Input: part model. Units: mm. Frame: model coordinates. Face numbers are marked on the shaded views. A direction names the side the tool comes from. Give positions to 0.01 mm unless a question says otherwise; leave off trailing zeros. Order: outer loops, then holes, each group sorted by start corner. A loop starts at its lowest first (then second) coordinate and runs counter-clockwise, first axis right, second up. Notation, with made-up numbers: (-4, 57) - (12, 57) arc R31 ccw to (12, 90) - close; hole circle Ø9 at (12.25, 57). An arc over 180 degrees is marked (long way). Answer in a Markdown table with one row per item. Add a question column.
1. Section query D-D on y = -0.4. Return loops of the section in (x, z), and give its area (3 significant figures).
2. Section query A-A on x = 0. Return loops of the section in (y, z).
3. Section query B-B on z = 0. Return loops of the section in (x, y), and give its area (3 significant figures).
4. Access query for the marked faces 1, 2, 3 and 4. Directions: +Z, -Z, +X, -X, +Y, -Y. A direction counts if a zero-diameter tool reaches every point of the face in a straight line with its end or side. Return the directions, or none.
5. Section query C-C on y = 1.95. Return loops of the section in (x, z).
6. Ray query, line 1 (Y direction, x = 0.5, z = -9.75); line 2 (X direction, y = 1.25, z = -2); line 3 (Z direction, x = 4.25, y = 1.3). Return the intervals inside material, ascending. Write a range as [from, to].
7. Contact query for flat-ended pins moving along their axis: pin 1 (1.4 mm diameter, centred on x = -13.5, y = 1.5, fed in from -Z); pin 2 (2 mm diameter, centred on x = -10.5, z = 2.5, fed in from -Y). Output: stop coordinate, or through.
```python
from build123d import *

# Parameters (mm, degrees)
EXTRUDE_1_DEPTH = 2.83
SKETCH_2_R      = 7.92
EXTRUDE_2_DEPTH = 1.5


with BuildPart() as part:
    # 草图1 → 凸台-拉伸1 (new body)
    with BuildSketch(Plane(origin=(0, 0, 0), x_dir=(1, 0, 0), z_dir=(0, 1, 0))):
        with BuildLine():
            Line((-16, 3.9), (-10.818502669, 3.9))
            ThreePointArc((-10.818502669, 3.9), (11.5, 0), (-10.818502669, -3.9))
            Line((-10.818502669, -3.9), (-16, -3.9))
            Line((-16, -3.9), (-16, 3.9))
        make_face()
    extrude(amount=EXTRUDE_1_DEPTH)

    # 草图2 → 凸台-拉伸2 (add)
    with BuildSketch(Plane.XZ):
        Circle(SKETCH_2_R)
    extrude(amount=EXTRUDE_2_DEPTH)


solid = part.part
```
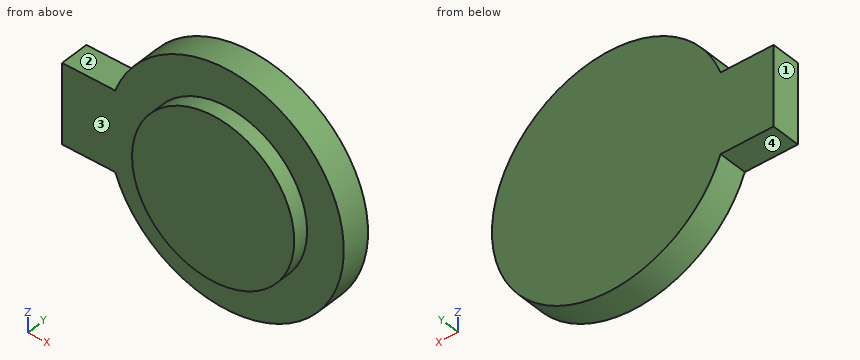
Answer:
| question | item | result |
|---|---|---|
| 1 | outline | circle Ø15.84 at (0, 0) |
| 1 | area | 197 mm² |
| 2 | outline | (-1.5, -7.92) - (0, -7.92) - (0, -11.5) - (2.83, -11.5) - (2.83, 11.5) - (0, 11.5) - (0, 7.92) - (-1.5, 7.92) - close |
| 3 | outline | (-16, 0) - (-7.92, 0) - (-7.92, -1.5) - (7.92, -1.5) - (7.92, 0) - (11.5, 0) - (11.5, 2.83) - (-16, 2.83) - close |
| 3 | area | 102 mm² |
| 4 | face 1 | +Z, -Z, -X, +Y, -Y |
| 4 | face 2 | +Z, -X, +Y, -Y |
| 4 | face 3 | -Y |
| 4 | face 4 | -Z, -X, +Y, -Y |
| 5 | outline | (-16, -3.9) - (-10.82, -3.9) arc R11.5 ccw (long way) to (-10.82, 3.9) - (-16, 3.9) - close |
| 6 | line 1 | y = [0, 2.83] |
| 6 | line 2 | x = [-16, 11.32] |
| 6 | line 3 | z = [-10.69, 10.69] |
| 7 | pin 1 | stops at z = -3.9 |
| 7 | pin 2 | stops at y = 0 |
